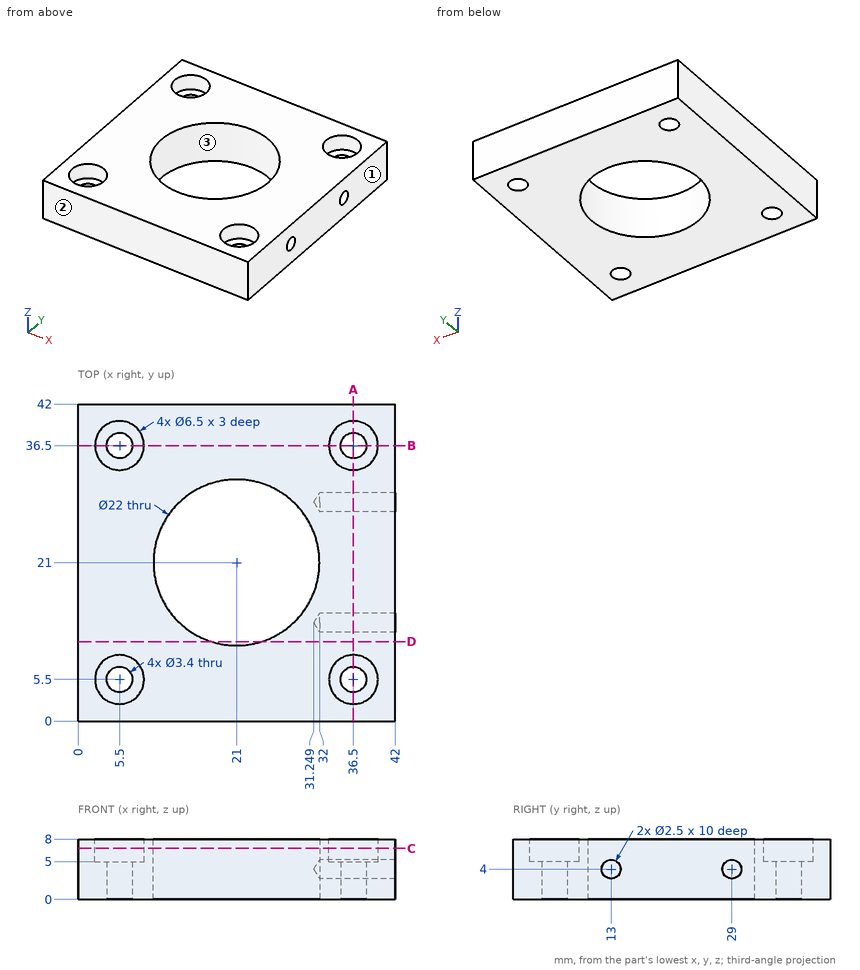
Could you check a few things on this drawing? It's one solid part, dimensions in mm from its lowest x, y, z. Coordinates: 2 decimals unless noted, no trailing zeros. Order: outer loops, then holes, each group sorted by start corner. A loop starts at its lowest first (then second) coordinate and runs counter-clockwise, first axis right, second up. Notation, with made-up numbers: M -16.75,72.25 L 20.25,72.25 A22 ccw 20.25,110.25 Z; hole C 40.5,12 d1. An arc over 180 degrees is marked long. Use one line per item in the form item = value. Start each with the question number.
1. Suppose I cut it at C-C on z = 6.75. Write out the boundary of the cut face in (x, y), then the cut area to 3 significant figures.
2. We'd pull the mould along Y, two halves only. Please class the marked faces 1, 2 and 3: +Y half, -Y half, draft (parallel to the pull), parting line (faces both ways), or undercut.
3. Please list where these lines run through material, in increasing order: line 1 (X direction, y = 5.5, z = 3.9); line 2 (Y direction, x = 39.5, z = 4).
4. Suppose I cut it at D-D on y = 10.5. Write out the boundary of the cut face in (x, z), then the cut area to 3 significant figures.
5. Suppose I cut it at B-B on y = 36.5. Write out the boundary of the cut face in (x, z).
6. For pin 1 (3 mm diameter, centred on x = 36.5, y = 36.5, fed in from +Z); pin 2 (5 mm diameter, centred on x = 36.5, y = 36.5, fed in from +Z), each with a flat end and sliding along its axis, tell me the tip position at first contact or that it passes through.
7. Suppose I cut it at A-A on x = 36.5. Write out the boundary of the cut face in (y, z).
Geometry says:
q1.outline = M 0,0 L 42,0 L 42,42 L 0,42 Z; hole C 5.5,5.5 d6.5; hole C 5.5,36.5 d6.5; hole C 21,21 d22; hole C 36.5,5.5 d6.5; hole C 36.5,36.5 d6.5
q1.area = 1,250 mm^2
q2.face_1 = draft
q2.face_2 = -Y half
q2.face_3 = undercut
q3.line_1 = 0 to 3.8, 7.2 to 34.8, 38.2 to 42
q3.line_2 = 0 to 11.75, 14.25 to 27.75, 30.25 to 42
q4.outline = M 0,0 L 17.72,0 L 17.72,8 L 0,8 Z; M 24.28,0 L 42,0 L 42,8 L 24.28,8 Z
q4.area = 284 mm^2
q5.outline = M 0,0 L 3.8,0 L 3.8,5 L 2.25,5 L 2.25,8 L 0,8 Z; M 7.2,0 L 34.8,0 L 34.8,5 L 33.25,5 L 33.25,8 L 8.75,8 L 8.75,5 L 7.2,5 Z; M 38.2,0 L 42,0 L 42,8 L 39.75,8 L 39.75,5 L 38.2,5 Z
q6.pin_1 = through
q6.pin_2 = 5
q7.outline = M 0,0 L 3.8,0 L 3.8,5 L 2.25,5 L 2.25,8 L 0,8 Z; M 7.2,0 L 34.8,0 L 34.8,5 L 33.25,5 L 33.25,8 L 8.75,8 L 8.75,5 L 7.2,5 Z; M 38.2,0 L 42,0 L 42,8 L 39.75,8 L 39.75,5 L 38.2,5 Z; hole C 13,4 d2.5; hole C 29,4 d2.5
